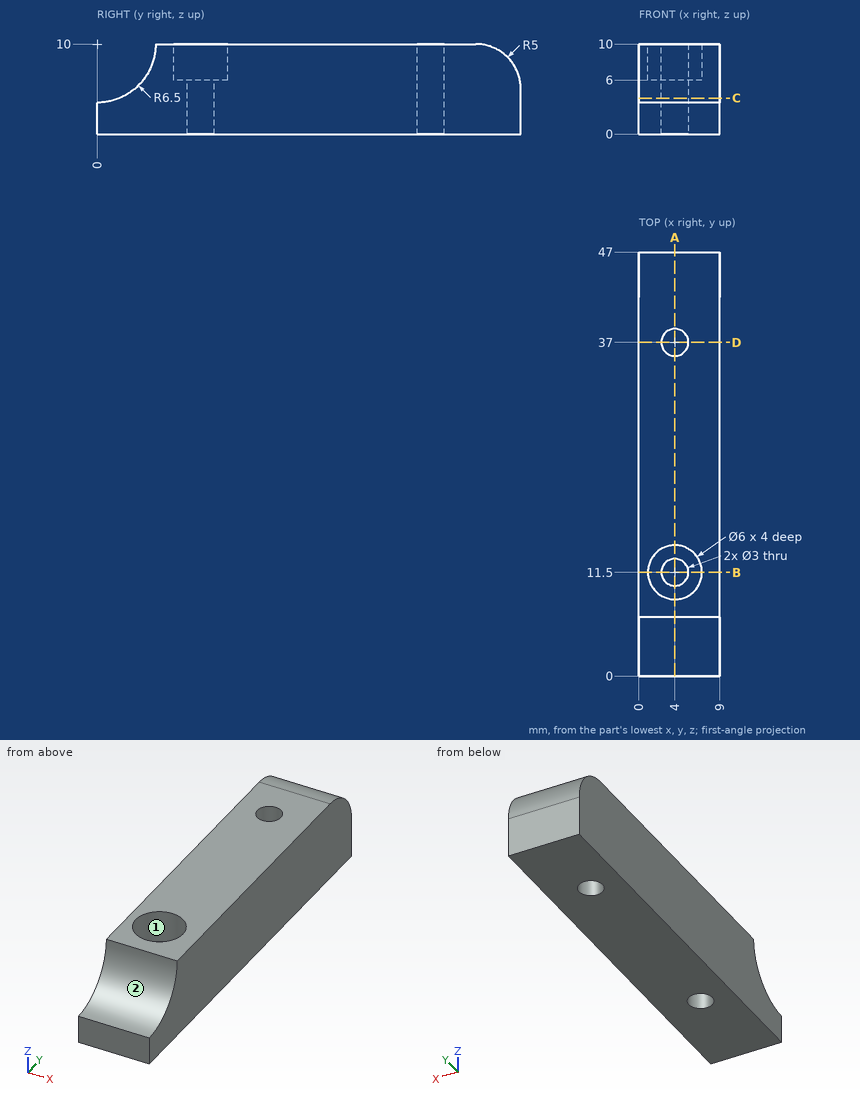
Geometry check sheet. Reference: drawing and pictorial views, mm from the part's lowest x, y, z. A direction names the side the tool comes from. Coordinates: 2 decimals unless noted, no trailing zeros. Write each loop counter-clockwise with the first axis right and the second up, starting at its lowest first coordinate (ties: lowest second). Pieces come first, ordered by that corner, then holes. Notation, with made-up numbers: M -30,5.5 L 3,5.5 A19 ccw 3,39.5 Z; hole C 35,15 d7. An arc over 180 degrees is marked long. Write item = value, one per line. Start each with the question number.
1. Go/stop test with flat-tipped pins: pin 1 (4 mm diameter, centred on x = 5.5, y = 20.5, fed in from -Z); pin 2 (2.5 mm diameter, centred on x = 4, y = 11.5, fed in from +Z); pin 3 (1.5 mm diameter, centred on x = 1, z = 7, fed in from -Y). Record where each tip stops, or that it passes through.
2. Sectioned sample at B-B (y = 11.5). Record the cut outline in (x, z), then the cut area to 3 significant figures.
3. Sectioned sample at A-A (x = 4). Record the cut outline in (y, z), then the cut area to 3 significant figures.
4. Thickness scan on probe 1 along Y at (x, z) = (4, 7.15); probe 2 along Y at (x, z) = (3, 3.25); probe 3 along X at (y, z) = (13.5, 7). Record the ranges inside material, lowest first.
5. Sectioned sample at C-C (z = 4). Record the cut outline in (x, y), then the cut area to 3 significant figures.
6. Tool access check on the marked faces 1 and 2. Record the directions out of +Z, -Z, +X, -X, +Y, -Y that give a thin tool (end or side, any length) a straight path to the whole face; none if there is none.
7. Sectioned sample at D-D (y = 37). Record the cut outline in (x, z).
The answers:
q1.pin_1 = 0
q1.pin_2 = through
q1.pin_3 = 5.31
q2.outline = M 0,0 L 2.5,0 L 2.5,6 L 1,6 L 1,10 L 0,10 Z; M 5.5,0 L 9,0 L 9,10 L 7,10 L 7,6 L 5.5,6 Z
q2.area = 48.0 mm²
q3.outline = M 0,0 L 10,0 L 10,6 L 8.5,6 L 8.5,10 L 6.5,10 A6.5 cw 0,3.5 Z; M 13,0 L 35.5,0 L 35.5,10 L 14.5,10 L 14.5,6 L 13,6 Z; M 38.5,0 L 47,0 L 47,5 A5 ccw 42,10 L 38.5,10 Z
q3.area = 359 mm²
q4.probe_1 = 5.84 to 8.5, 14.5 to 35.5, 38.5 to 46.51
q4.probe_2 = 0 to 10.38, 12.62 to 35.88, 38.12 to 47
q4.probe_3 = 0 to 1.76, 6.24 to 9
q5.outline = M 0,2.5 L 9,2.5 L 9,47 L 0,47 Z; hole C 4,11.5 d3; hole C 4,37 d3
q5.area = 386 mm²
q6.face_1 = +Z
q6.face_2 = +Z, +X, -X, -Y
q7.outline = M 0,0 L 2.5,0 L 2.5,10 L 0,10 Z; M 5.5,0 L 9,0 L 9,10 L 5.5,10 Z
